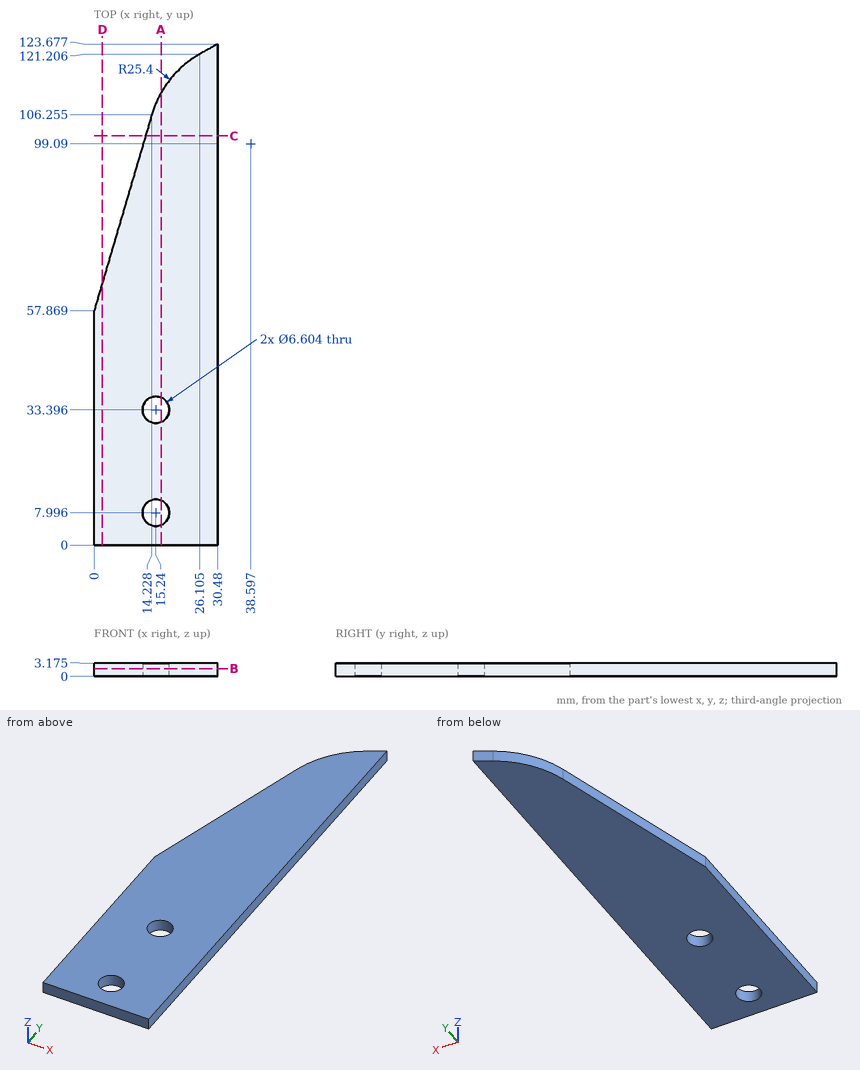
Could you check a few things on this drawing? It's one solid part, dimensions in mm from its lowest x, y, z. Give positions to 0.01 mm unless a question says otherwise; leave off trailing zeros. Order: outer loops, then holes, each group sorted by start corner. A loop starts at its lowest first (then second) coordinate and runs counter-clockwise, first axis right, second up.
1. I need wall thicknesses on L1, parallel to Y at x = 15.24, z = 2 (1 decimal); L2, parallel to X at y = 7.5, z = 2.05 (1 decimal); L3, parallel to X at y = 7, z = 1.65. Which ranges of each line are inside material? Lowest first, please.
Answers below:
L1: y = 0 to 4.7, 11.3 to 30.1, 36.7 to 109.1
L2: x = 0 to 12, 18.5 to 30.5
L3: x = 0 to 12.09, 18.39 to 30.48
2. Suppose I cut it at A-A (x = 16.5). Write out the boundary of the cut face in (y, z) (1 decimal).
Answers below:
outline: (0, 0) - (4.9, 0) - (4.9, 3.2) - (0, 3.2) - close; (11, 0) - (30.3, 0) - (30.3, 3.2) - (11, 3.2) - close; (36.4, 0) - (111.6, 0) - (111.6, 3.2) - (36.4, 3.2) - close
3. Suppose I cut it at C-C (y = 101). Write out the boundary of the cut face in (x, z) (1 decimal).
Answers below:
outline: (12.7, 0) - (30.5, 0) - (30.5, 3.2) - (12.7, 3.2) - close
4. Suppose I cut it at B-B (z = 1.8). Write out the boundary of the cut face in (x, y) (1 decimal).
Answers below:
outline: (0, 0) - (30.5, 0) - (30.5, 123.7) - (26.1, 121.2) arc R25.4 ccw to (14.2, 106.3) - (0, 57.9) - close; hole circle Ø6.6 at (15.2, 8); hole circle Ø6.6 at (15.2, 33.4)
5. Suppose I cut it at D-D (x = 2). Write out the boundary of the cut face in (y, z) (1 decimal).
Answers below:
outline: (0, 0) - (64.7, 0) - (64.7, 3.2) - (0, 3.2) - close
